from build123d import *

# Parameters (mm, degrees)
EXTRUDE_1_DEPTH = 45
SKETCH_2_W      = 1
SKETCH_2_H      = 1.5
SKETCH_3_W      = 10
SKETCH_3_H      = 28
EXTRUDE_2_DEPTH = 0.1


with BuildPart() as part:
    # Эскиз1 → Бобышка-Вытянуть1 (new body)
    with BuildSketch(Plane.XY):
        with BuildLine():
            Line((-5, 3.31662479), (5, 3.31662479))
            ThreePointArc((5, 3.31662479), (0, -6), (-5, 3.31662479))
        make_face()
    extrude(amount=EXTRUDE_1_DEPTH)

    # Эскиз2 → Вырез-Повернуть1 (revolve, cut)
    with BuildSketch(Plane(origin=(0, 0, 0), x_dir=(1, 0, 0), z_dir=(0, 1, 0))):
        with Locations((5.5, -16.25)):
            Rectangle(SKETCH_2_W, SKETCH_2_H)
    revolve(axis=Axis((0, 0, 1000), (0, 0, -1)), mode=Mode.SUBTRACT)

    # Зеркальное отражение1: part across plane


with BuildPart() as part_1:
    add(part.part)
    add(part.part.mirror(Plane.XY))

    # Эскиз3 → Бобышка-Вытянуть2 (add)
    with BuildSketch(Plane(origin=(0, 3.31662479, 0), x_dir=(1, 0, 0), z_dir=(0, 1, 0))):
        with Locations((0, -31)):
            Rectangle(SKETCH_3_W, SKETCH_3_H)
    extrude(amount=EXTRUDE_2_DEPTH)


solid = part_1.part
Could you check a few things on this model? Use its own coordinates, in mm. A direction names the side the tool comes from. Coordinates: 2 decimals unless noted, no trailing zeros. Order: outer loops, then holes, each group sorted by start corner. A loop starts at its lowest first (then second) coordinate and runs counter-clockwise, first axis right, second up. Notation, with made-up numbers: (78, 29) -> (107, 29) arc R16 cw to (107, 52) -> close; hole circle Ø5 at (0.5, -14). An arc over 180 degrees is marked (long way). One line per question, with ' | ' between items.
Q1. I'm going to push flat-ended pins straight in: P1, Ø1, axis at y = -3.5, z = 3, coming from the +X side; P2, Ø1, axis at x = -3, z = 0.5, coming from the +Y side; P3, Ø1, axis at y = 1, z = 2.5, coming from the +X side. Where does each tip first touch, or does it pass through?
Return value:
P1: x = 5.2 | P2: y = 3.32 | P3: x = 5.98
Q2. Imagine slicing it at D-D on z = -25.5. Please give me the cut outline in (x, y), and give its area (3 significant figures).
Return value:
outline: (-5, 3.32) arc R6 ccw (long way) to (5, 3.32) -> close | area: 94.2 mm²
Q3. On a 3-axis mill with a long thin cutter (end or side, diameter ignored), from which of +Z, -Z, +X, -X, +Y, -Y can I reach the whole of each face in a straight line? I mean faces 5 (the face through (0, 3.417, 31)), 6 (the face through (0, 3.317, -14)), 7 (the face through (0, -5, 16)). Say none if no direction works.
Return value:
face 5: +Z, -Z, +X, -X, +Y | face 6: -Z, +X, -X, +Y | face 7: none
Q4. If I drill on L1, parallel to Z at x = 4.25, y = -3; L2, parallel to Y at x = 0, z = -7; L3, parallel to X at y = -0.25, z = 32.5, over which ranges is the centre line in solid material (lowest first)?
Return value:
L1: -45 to -17, -15.5 to 15.5, 17 to 45 | L2: -6 to 3.32 | L3: -5.99 to 5.99
Q5. Thinking about a two-plate mould opening in Z: for faces 1 (the face through (0, -1, -45)), 2 (the face through (0, -1, 45)), 3 (the face through (0, -6, 0)), 4 (the face through (0.5, -5.2, -15.5)), which applies, pulls with the +Z half, pulls with the -Z half, needs draft (parallel to the pull), parting line crosses it, or undercut?
Return value:
face 1: pulls with the -Z half | face 2: pulls with the +Z half | face 3: needs draft | face 4: undercut
Q6. Imagine slicing it at A-A on x = -1.5. Please give me the cut outline in (y, z).
Return value:
outline: (-5.81, -45) -> (3.32, -45) -> (3.32, 17) -> (3.42, 17) -> (3.42, 45) -> (-5.81, 45) -> (-5.81, 17) -> (-4.77, 17) -> (-4.77, 15.5) -> (-5.81, 15.5) -> (-5.81, -15.5) -> (-4.77, -15.5) -> (-4.77, -17) -> (-5.81, -17) -> close
Q7. Imagine slicing it at B-B on z = 18. Please give me the cut outline in (x, y), and give its area (3 significant figures).
Return value:
outline: (-5, 3.32) arc R6 ccw (long way) to (5, 3.32) -> (5, 3.42) -> (-5, 3.42) -> close | area: 95.2 mm²
Q8. Imagine slicing it at C-C on y = -2. Please give me the cut outline in (x, z).
Return value:
outline: (-5.66, -45) -> (5.66, -45) -> (5.66, -17) -> (4.58, -17) -> (4.58, -15.5) -> (5.66, -15.5) -> (5.66, 15.5) -> (4.58, 15.5) -> (4.58, 17) -> (5.66, 17) -> (5.66, 45) -> (-5.66, 45) -> (-5.66, 17) -> (-4.58, 17) -> (-4.58, 15.5) -> (-5.66, 15.5) -> (-5.66, -15.5) -> (-4.58, -15.5) -> (-4.58, -17) -> (-5.66, -17) -> close
